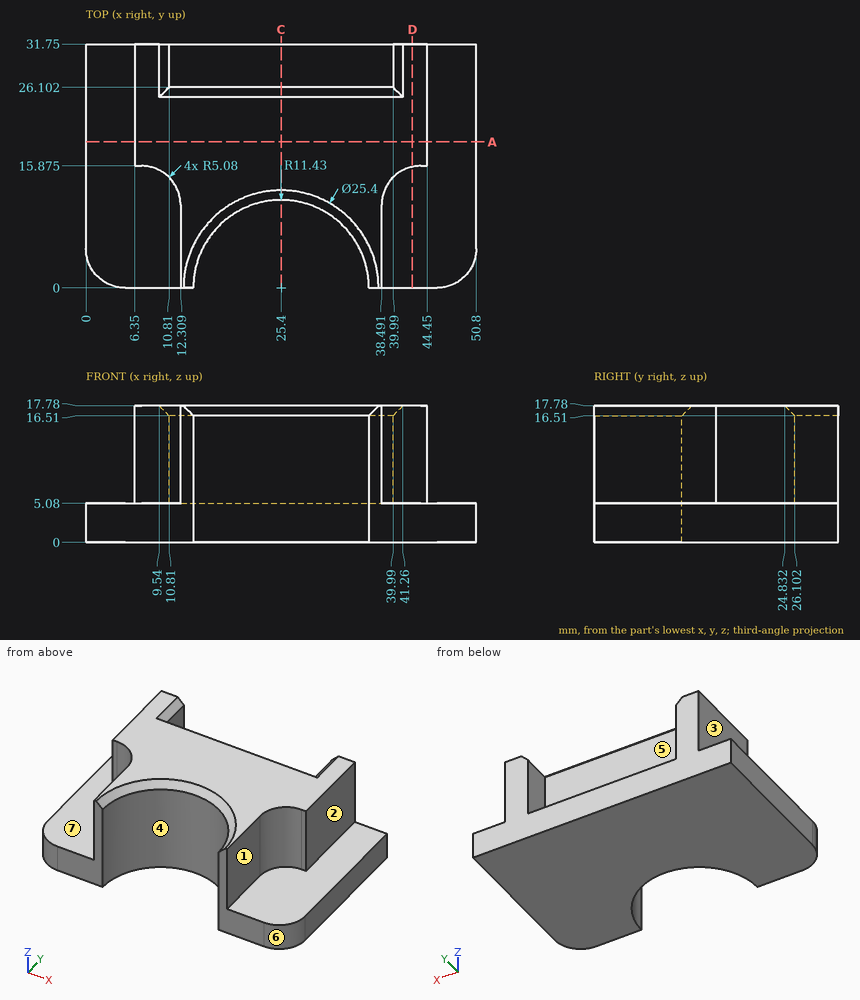
Drawing for the job (mm, zero at the part's lowest x, y, z). A direction names the side the tool comes from. Round coordinates to 2 decimals unless told otherwise and drop trailing zeros. Order: outer loops, then holes, each group sorted by start corner. A loop starts at its lowest first (then second) coordinate and runs counter-clockwise, first axis right, second up. Notation, with made-up numbers: (55.5, 77) -> (93.5, 77) arc R7 cw to (93.5, 86) -> close; hole circle Ø10 at (59, 80.5). An arc over 180 degrees is marked (long way). Write item = value, one per line. Start each with the question number.
(1) Pull direction X, two halves, no side cores. Call the marked faces 4, 5, 6 and 7: released by +X, released by -X, zero draft, split by the parting line, or undercut.
(2) Pin check, flat tips, straight feed: P1, Ø8.5, axis at y = 7.5, z = 11, coming from the -X side; P2, Ø5, axis at x = 22, y = 5.5, coming from the -Z side; P3, Ø3, axis at y = 3, z = 13.5, coming from the +X side; P4, Ø3, axis at x = 21, y = 30.5, coming from the +Z side. Stop position of each tip, or through.
(3) Probe line 1 (X direction, y = 30, z = 8); line 2 (Z direction, x = 11, y = 10); line 3 (X direction, y = 17, z = 7.25). List the from-to ranges inside material, lowest first. Write a range as [from, to].
(4) Cut at A-A, the plane y = 19. List the corners of the cut face in (x, z).
(5) Which spindle directions (+Z, -Z, +X, -X, +Y, -Y) get a long thin tool onto all of the face, cutting with end or side? Do the marked faces 1, 2 and 3. Say none if no direction does.
(6) Cut at D-D, the plane x = 42.5. List the corners of the cut face in (y, z).
(7) Cut at C-C, the plane x = 25.4. List the corners of the cut face in (y, z), then the cut area to 3 significant figures.
Model answer:
q1.face_4 = undercut
q1.face_5 = undercut
q1.face_6 = released by +X
q1.face_7 = zero draft
q2.P1 = 12.22
q2.P2 = through
q2.P3 = 38.49
q2.P4 = 5.08
q3.line_1 = [6.35, 10.81], [39.99, 44.45]
q3.line_2 = [0, 5.08]
q3.line_3 = [6.35, 44.45]
q4.outline = (0, 0) -> (50.8, 0) -> (50.8, 5.08) -> (44.45, 5.08) -> (44.45, 17.78) -> (6.35, 17.78) -> (6.35, 5.08) -> (0, 5.08) -> close
q5.face_1 = +Z, +X, -Y
q5.face_2 = +Z, +X, +Y, -Y
q5.face_3 = +Z, -X, +Y, -Y
q6.outline = (0, 0) -> (31.75, 0) -> (31.75, 17.78) -> (15.76, 17.78) -> (15.76, 5.08) -> (0, 5.08) -> close
q7.outline = (11.43, 0) -> (31.75, 0) -> (31.75, 5.08) -> (26.1, 5.08) -> (26.1, 16.51) -> (24.83, 17.78) -> (12.7, 17.78) -> (11.43, 16.51) -> close
q7.area = 288 mm2
